Could you check a few things on this model? Use its own coordinates, in mm. Face numbers are marked on the shaded views. A direction names the side the tool comes from. Round coordinates to 2 decimals unless told otherwise and drop trailing zeros. Loops run counter-clockwise (first coordinate to the right, second up) from the corner with the lowest first, then second, coordinate; pieces in that order, holes last.
from build123d import *

# Parameters (mm, degrees)
BOSS_EXTRUDE1_DEPTH = 20
SKETCH2_W           = 1
SKETCH2_H           = 2.5
SKETCH2_H_2         = 10
BOSS_EXTRUDE2_DEPTH = 2.5
SKETCH2_3_R         = 2.5
CUT_EXTRUDE1_DEPTH  = 35.641016151
SKETCH3_W           = 1
SKETCH3_H           = 10
BOSS_EXTRUDE3_DEPTH = 2.5
SKETCH5_R           = 6
CUT_EXTRUDE3_DEPTH  = 17
SKETCH7_R           = 6
CUT_EXTRUDE5_DEPTH  = 17


with BuildPart() as part:
    # Sketch1 → Boss-Extrude1 (new body)
    with BuildSketch(Plane(origin=(0, 0, 0), x_dir=(1, 0, 0), z_dir=(0, 1, 0))):
        Polygon((0, 7.5), (3, 7.5), (3, 12.5), (0, 12.5), (0, 20), (20, 20), (20, 0), (0, 0), align=None)
    extrude(amount=BOSS_EXTRUDE1_DEPTH)

    # Sketch2 → Boss-Extrude2 (add)
    with BuildSketch(Plane(origin=(0, 20, 0), x_dir=(1, 0, 0), z_dir=(0, 1, 0))):
        with Locations((2.5, 6.25)):
            Rectangle(SKETCH2_W, SKETCH2_H)
        with Locations((2.5, 13.75)):
            Rectangle(SKETCH2_W, SKETCH2_H)
        with Locations((17.5, 10)):
            Rectangle(SKETCH2_W, SKETCH2_H_2)
    extrude(amount=BOSS_EXTRUDE2_DEPTH)

    # Sketch2<3> → Cut-Extrude1 (cut, through all)
    with BuildSketch(Plane(origin=(0, 20, 0), x_dir=(1, 0, 0), z_dir=(0, 1, 0))):
        with Locations(Location((10, 10, 0), (0, 0, 270))):
            Circle(SKETCH2_3_R)
    extrude(amount=-CUT_EXTRUDE1_DEPTH, mode=Mode.SUBTRACT)

    # Sketch3 → Boss-Extrude3 (add)
    with BuildSketch(Plane.ZY):
        with Locations((-2.5, 10)):
            Rectangle(SKETCH3_W, SKETCH3_H)
        with Locations((-17.5, 10)):
            Rectangle(SKETCH3_W, SKETCH3_H)
    extrude(amount=BOSS_EXTRUDE3_DEPTH)

    # Sketch5 → Cut-Extrude3 (cut)
    with BuildSketch(Plane(origin=(20, 0, 0), x_dir=(0, 0, -1), z_dir=(1, 0, 0))):
        with Locations((10, 10)):
            Circle(SKETCH5_R)
    extrude(amount=-CUT_EXTRUDE3_DEPTH, mode=Mode.SUBTRACT)

    # Sketch7 → Cut-Extrude5 (cut)
    with BuildSketch(Plane.XZ):
        with Locations(Location((10, -10, 0), (0, 0, 270))):
            Circle(SKETCH7_R)
    extrude(amount=-CUT_EXTRUDE5_DEPTH, mode=Mode.SUBTRACT)


solid = part.part
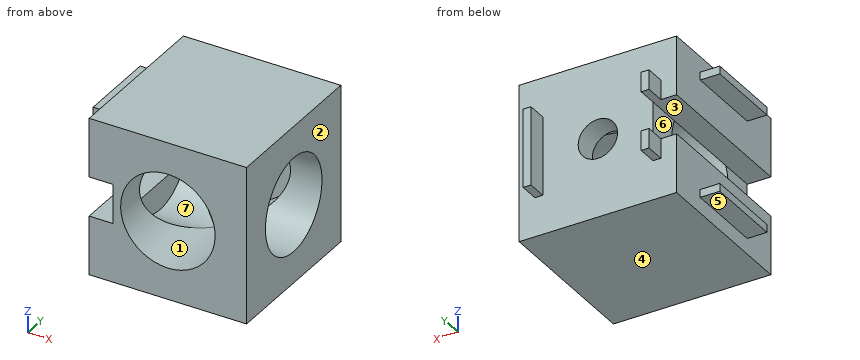
Item 1: If we section it at C-C, the plane z = -6.5: Please give me the cut outline in (x, y).
Results list:
outline: (0, 0) - (5.13, 0) - (5.13, 5.13) - (3, 5.13) - (3, 14.87) - (5.13, 14.87) - (5.13, 17) - (14.87, 17) - (14.87, 14.87) - (20, 14.87) - (20, 20) - (18, 20) - (18, 22.5) - (17, 22.5) - (17, 20) - (3, 20) - (3, 22.5) - (2, 22.5) - (2, 20) - (0, 20) - close; (14.87, 0) - (20, 0) - (20, 5.13) - (14.87, 5.13) - close
Item 2: For the marked faces 4, 5, 6 and 7, which set-ups out of +Z, -Z, +X, -X, +Y, -Y let a thin tool reach every point of the face, with its end or its side?
Results list:
face 4: -Z, +X, -X, +Y, -Y
face 5: -Z, -X, +Y, -Y
face 6: -X, +Y, -Y
face 7: +X
Item 3: Will these pins go through, and if not, where does the flat tip stop? pin 1 (8 mm diameter, centred on y = 9, z = -12, fed in from -X); pin 2 (1 mm diameter, centred on x = 12, z = -5, fed in from +Y); pin 3 (1.2 mm diameter, centred on x = -1.5, y = 12, fed in from -Z).
Results list:
pin 1: stops at x = 0
pin 2: stops at y = 20
pin 3: stops at z = -18
Item 4: If we section it at B-B, the plane y = 2.5: Please give me the cut outline in (x, z), then the cut area to 3 significant figures.
Results list:
outline: (0, -20) - (20, -20) - (20, 0) - (0, 0) - (0, -7.5) - (3, -7.5) - (3, -12.5) - (0, -12.5) - close; hole circle Ø12 at (10, -10)
area: 272 mm2
Item 5: We'd pull the mould along X, two halves only. Please class the marked faces 1, 2 and 3: released by +X, released by -X, zero draft, split by the parting line, or undercut.
Results list:
face 1: undercut
face 2: released by +X
face 3: zero draft
Item 6: If we section it at D-D, the plane y = 14: Please give me the cut outline in (x, z), then the cut area to 3 significant figures.
Results list:
outline: (-2.5, -18) - (0, -18) - (0, -20) - (20, -20) - (20, -14.47) - (14, -14.47) arc R6 cw to (6, -14.47) - (3, -14.47) - (3, -12.5) - (0, -12.5) - (0, -17) - (-2.5, -17) - close; (-2.5, -3) - (0, -3) - (0, -7.5) - (3, -7.5) - (3, -5.53) - (6, -5.53) arc R6 cw to (14, -5.53) - (20, -5.53) - (20, 0) - (0, 0) - (0, -2) - (-2.5, -2) - close
area: 221 mm2
Item 7: If I drill on line 1 along Z through (x, y) = (10, 6); line 2 along X through (y, z) = (18.9, -10); line 3 along Z through (x, y) = (-1, 7.5), over which ranges is the centre line in solid material (lowest first)?
Results list:
line 1: z = -20 to -16, -4 to 0
line 2: x = 3 to 7.5, 12.5 to 20
line 3: z = -18 to -17, -3 to -2
Item 8: If we section it at A-A, the plane z = -10: Please give me the cut outline in (x, y), then the cut area to 3 significant figures.
Results list:
outline: (3, 0) - (4, 0) - (4, 4) - (3, 4) - close; (3, 16) - (4, 16) - (4, 17) - (7.5, 17) - (7.5, 20) - (3, 20) - close; (12.5, 17) - (16, 17) - (16, 16) - (20, 16) - (20, 20) - (18, 20) - (18, 22.5) - (17, 22.5) - (17, 20) - (12.5, 20) - close; (16, 0) - (20, 0) - (20, 4) - (16, 4) - close
area: 63.5 mm2
